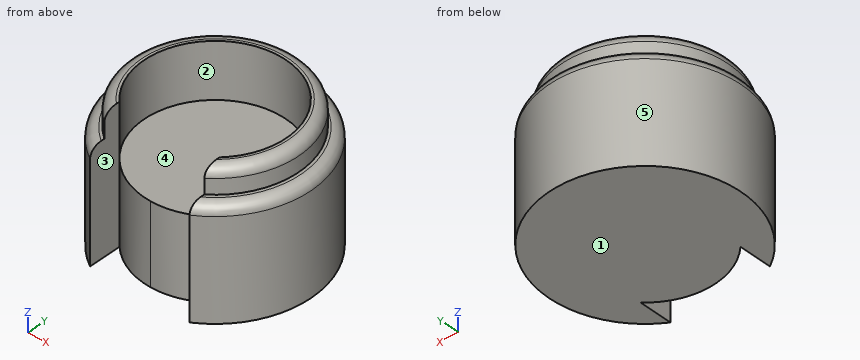
from build123d import *

# Parameters (mm, degrees)
F0_R     = 48.41875
F1_DEPTH = 55.5625
F2_R     = 42.06875
F3_DEPTH = 12.7
F4_R     = 35.71875
F5_DEPTH = 27.78125
F6_R     = 5.08
F8_DEPTH = 100.076


with BuildPart() as f1:
    # F0 (on Top) → F1 (new body)
    with BuildSketch(Plane.XY):
        with Locations((0.225817, -0.361804)):
            Circle(F0_R)
    extrude(amount=F1_DEPTH)

    # F2 (on face) → F3 (join)
    with BuildSketch(Plane.XY.offset(55.5625)):
        Circle(F2_R)
    extrude(amount=F3_DEPTH)

    # F4 (on face) → F5 (cut)
    with BuildSketch(Plane.XY.offset(68.2625)):
        Circle(F4_R)
    extrude(amount=-F5_DEPTH, mode=Mode.SUBTRACT)

    # F6
    f6_edges = [f1.edges().sort_by_distance(p)[0] for p in [
        (-48.192933, -0.361804, 55.5625),
        (-42.06875, 0, 68.2625),
    ]]
    fillet(f6_edges, radius=F6_R)

    # F7 (on Top) → F8 (cut)
    with BuildSketch(Plane.XY):
        with BuildLine():
            Line((25.284194, -55.836208), (25.284194, -25.229717))
            ThreePointArc((25.284194, -25.229717), (13.686766, -32.992447), (0, -35.71875))
            Line((0, -35.71875), (0, -55.836208))
            Line((0, -55.836208), (25.284194, -55.836208))
        make_face()
        with BuildLine():
            ThreePointArc((0, -35.71875), (-13.686766, -32.992447), (-25.284194, -25.229717))
            Line((-25.284194, -25.229717), (-25.284194, -55.836208))
            Line((-25.284194, -55.836208), (0, -55.836208))
            Line((0, -55.836208), (0, -35.71875))
        make_face()
    extrude(amount=F8_DEPTH, mode=Mode.SUBTRACT)


solid = f1.part
Work out the finished part from the listing and answer in its coordinate system (mm). Face numbers are marked on the shaded views. A direction names the side the tool comes from. Give positions to 0.01 mm unless a question says otherwise; leave off trailing zeros. Order: outer loops, then holes, each group sorted by start corner. A loop starts at its lowest first (then second) coordinate and runs counter-clockwise, first axis right, second up. Notation, with made-up numbers: (-27, 59) -> (32, 59) arc R22 cw to (32, 84) -> close; hole circle Ø9 at (66, 87.5). An arc over 180 degrees is marked (long way). Answer as a JSON object with one key per item and string values. Group by question number.
1. The mould has two halves that part along Y. Classify the marked faces 3, 4 and 5: released by +Y, released by -Y, zero draft, split by the parting line, or undercut.
2. Consider line 1 along X through (y, z) = (0, 62); line 2 along Z through (x, y) = (17, -2); line 3 along Z through (x, y) = (38.5, 21). Determine where each line is inside the solid, lowest interval first. Write a range as [from, to].
3. Section B-B on z = 42.5 is taken. Determine the outline of the cut face in (x, y), plus the area to 3 significant figures.
4. A tool of negligible diameter and unlimited length cuts with its end or side. For the marked faces 1 and 2, from which of +Z, -Z, +X, -X, +Y, -Y can it reach the whole face along a straight path? Write none if from no direction.
5. Section A-A on z = 28 is taken. Determine the outline of the cut face in (x, y).
6. Flat-ended cylindrical pins translate along their axes: pin 1 Ø18 at (y, z) = (-31.5, 26.5) entering from -X; pin 2 Ø1 at (x, z) = (-12, 25.5) entering from +Y; pin 3 Ø4 at (y, z) = (29, 28) entering from +X; pin 4 Ø3 at (x, y) = (20.5, 38.5) entering from -Z. Find the tip coordinate at first contact, or state that the pin passes through.
Result sheet:
{
 "1": {"face 3": "zero draft", "face 4": "undercut", "face 5": "split by the parting line"},
 "2": {"line 1": "x = [-42.07, -35.72], [35.72, 42.07]", "line 2": "z = [0, 40.48]", "line 3": "z = [0, 55.54]"},
 "3": {"outline": "(-25.28, -41.52) -> (-25.28, -25.23) arc R35.72 cw (long way) to (25.28, -25.23) -> (25.28, -41.79) arc R48.42 ccw (long way) to start", "area": "2,650 mm^2"},
 "4": {"face 1": "-Z, +X, -X, +Y, -Y", "face 2": "+Z"},
 "5": {"outline": "(-25.28, -41.52) -> (-25.28, -25.23) arc R35.72 ccw to (0, -35.72) arc R35.72 ccw to (25.28, -25.23) -> (25.28, -41.79) arc R48.42 ccw (long way) to start"},
 "6": {"pin 1": "stops at x = -42.84", "pin 2": "stops at y = 46.62", "pin 3": "stops at x = 40.17", "pin 4": "stops at z = 0"}
}
